Could you check a few things on this model? Use its own coordinates, in mm. A direction names the side the tool comes from. Give positions to 0.01 mm unless a question says otherwise; leave off trailing zeros. Loops run counter-clockwise (first coordinate to the right, second up) from the corner with the lowest first, then second, coordinate; pieces in that order, holes last. Notation, with made-up numbers: (47.25, 34.5) - (61.25, 34.5) arc R36 ccw to (61.25, 72.5) - close; hole circle Ø10 at (5, 56). An arc over 180 degrees is marked (long way). One line per item, written item: value. Start each with the question number.
Q1. I'm going to push flat-ended pins straight in: P1, Ø18, axis at x = 1.5, y = 18.5, coming from the +Z side; P2, Ø0.8, axis at x = -79, y = 0.5, coming from the -Z side; P3, Ø5, axis at x = -66, z = 0, coming from the +Y side. Where does each tip first touch, or does it pass through?
Q2. I want a section at D-D (y = 7). Please give me the cut outline in (x, z), then the cut area to 3 significant figures.
Q3. For faces 1 (the face through (-1.306, 5.572, 58.065)), 2 (the face through (-1, 1, -1)), 3 (the face through (-94.5, 10.6, -55)), 4 (the face through (94.6, 10.6, -55)), 5 (the face through (-94, 20, 1)), which set-ups out of +Z, -Z, +X, -X, +Y, -Y let a thin tool reach every point of the face, with its end or its side?
Q4. I want a section at C-C (x = 66). Please give me the cut outline in (y, z).
Q5. I want a section at B-B (z = 50). Please give me the cut outline in (x, y), then the cut area to 3 significant figures.
Q6. If I drill on line 1 (X direction, y = 36, z = -18); line 2 (Y direction, x = -69, z = -4); line 3 (Z direction, x = 42, y = 36.5), over which ranges is the centre line in solid material (lowest first)? Write a range as from..to.
Q7. I want a section at A-A (y = 31.5). Please give me the cut outline in (x, z).
Q8. If we mould it in two halves opening along X, with no side actions, what happens to faces 6 (the face through (1, 20, -55.737)), 7 (the face through (-93.263, 5, 58)), 8 (the face through (82.41, 0.49, -52.38))? For each: released by +X, released by -X, zero draft, split by the parting line, or undercut.
```python
from build123d import *

# Parameters (mm, degrees)
SKETCH2_W                    = 190
SKETCH2_H                    = 110
BASE_FLANGE1_DEPTH           = 1
EDGE_FLANGE1_STRIP_W         = 5.4732
EDGE_FLANGE1_STRIP_H         = 1
EDGE_FLANGE1_STRIP_CUT_DEPTH = 110
EDGE_FLANGE1_DEPTH           = 110
SKETCH16_R                   = 2.25
CUT_EXTRUDE1_DEPTH           = 117.163677628
SKETCH17_W                   = 10
SKETCH17_H                   = 25
CUT_EXTRUDE2_DEPTH           = 117.163677628
EDGE_FLANGE2_DEPTH           = 142
EDGE_FLANGE3_DEPTH           = 186.5268
SKETCH29_R                   = 2.25
CUT_EXTRUDE3_DEPTH           = 204.225548722
SKETCH30_R                   = 2.25
CUT_EXTRUDE4_DEPTH           = 120.271218881


# Sheet-metal steps are written as plain solids
with BuildPart() as part:
    # Sketch2 → Base-Flange1 (new body)
    with BuildSketch(Plane(origin=(0, 0, 0), x_dir=(1, 0, 0), z_dir=(0, 1, 0))):
        Rectangle(SKETCH2_W, SKETCH2_H)
    extrude(amount=BASE_FLANGE1_DEPTH)

    # Edge-Flange1 strip (across the edge) → Edge-Flange1 strip cut (cut)
    with BuildSketch(Plane(origin=(95, 1, 55), x_dir=(-1, 0, 0), z_dir=(0, 0, -1))):
        with Locations((-1, -0.5)):
            Rectangle(EDGE_FLANGE1_STRIP_W, EDGE_FLANGE1_STRIP_H)
    edge_flange1_strip_cut = extrude(amount=EDGE_FLANGE1_STRIP_CUT_DEPTH, mode=Mode.SUBTRACT)

    # Edge-Flange1 section (across the edge) → Edge-Flange1 (add)
    with BuildSketch(Plane(origin=(95, 1, 55), x_dir=(-1, 0, 0), z_dir=(0, 0, -1))):
        with BuildLine():
            Line((0, 0.7366), (0, 37))
            Line((0, 37), (1, 37))
            Line((1, 37), (1, 0.7366))
            ThreePointArc((1, 0.7366), (1.215745145, 0.215745145), (1.7366, 0))
            Line((1.7366, 0), (1.7366, -1))
            ThreePointArc((1.7366, -1), (0.508638364, -0.491361636), (0, 0.7366))
        make_face()
    edge_flange1 = extrude(amount=EDGE_FLANGE1_DEPTH)

    # Mirror1: Edge-Flange1 strip cut, Edge-Flange1 across plane
    add(edge_flange1_strip_cut.mirror(Plane(origin=(0, 0, 0), x_dir=(0, 0, 1), z_dir=(1, 0, 0))), mode=Mode.SUBTRACT)
    add(edge_flange1.mirror(Plane(origin=(0, 0, 0), x_dir=(0, 0, 1), z_dir=(1, 0, 0))))

    # Sketch16 → Cut-Extrude1 (cut, through all)
    with BuildSketch(Plane.XZ):
        with Locations(Location((-55, 0, 0), (0, 0, 270))):
            Circle(SKETCH16_R)
        with Locations(Location((55, 0, 0), (0, 0, 270))):
            Circle(SKETCH16_R)
        with Locations(Location((66, 0, 0), (0, 0, 270))):
            Circle(SKETCH16_R)
        with Locations(Location((-66, 0, 0), (0, 0, 270))):
            Circle(SKETCH16_R)
    extrude(amount=-CUT_EXTRUDE1_DEPTH, mode=Mode.SUBTRACT)

    # Sketch17 → Cut-Extrude2 (cut, through all)
    with BuildSketch(Plane.XZ):
        with Locations((-79, 0)):
            Rectangle(SKETCH17_W, SKETCH17_H)
    cut_extrude2 = extrude(amount=-CUT_EXTRUDE2_DEPTH, mode=Mode.SUBTRACT)

    # Mirror2: Cut-Extrude2 across plane
    add(cut_extrude2.mirror(Plane(origin=(0, 0, 0), x_dir=(0, 0, 1), z_dir=(1, 0, 0))), mode=Mode.SUBTRACT)

    # Edge-Flange2 section (across the edge) → Edge-Flange2 (add)
    with BuildSketch(Plane(origin=(71, 1, -55.7366), x_dir=(0, 0, 1), z_dir=(-1, 0, 0))):
        with BuildLine():
            Line((-1, 0.7366), (-1, 37))
            Line((-1, 37), (0, 37))
            Line((0, 37), (0, 0.7366))
            ThreePointArc((0, 0.7366), (0.215745145, 0.215745145), (0.7366, 0))
            Line((0.7366, 0), (0.7366, -1))
            ThreePointArc((0.7366, -1), (-0.491361636, -0.491361636), (-1, 0.7366))
        make_face()
    extrude(amount=EDGE_FLANGE2_DEPTH)

    # Edge-Flange3 section (across the edge) → Edge-Flange3 (add)
    with BuildSketch(Plane(origin=(-93.2634, 1, 55.425276208), x_dir=(0, 0.5000000000000041, -0.8660254037844364), z_dir=(1, 0, 0))):
        with BuildLine():
            Line((-1, 0.425276208), (-1, 10))
            Line((-1, 10), (0, 10))
            Line((0, 10), (0, 0.425276208))
            ThreePointArc((0, 0.425276208), (0.098685688, 0.056976208), (0.3683, -0.212638104))
            Line((0.3683, -0.212638104), (-0.1317, -1.078663508))
            ThreePointArc((-0.1317, -1.078663508), (-0.767339716, -0.443023792), (-1, 0.425276208))
        make_face()
    extrude(amount=EDGE_FLANGE3_DEPTH)

    # Sketch29 → Cut-Extrude3 (cut, through all)
    with BuildSketch(Plane.ZY.offset(95)):
        with Locations(Location((50, 19.8683, 0), (0, 0, 270))):
            Circle(SKETCH29_R)
    extrude(amount=-CUT_EXTRUDE3_DEPTH, mode=Mode.SUBTRACT)

    # Sketch30 → Cut-Extrude4 (cut, through all)
    with BuildSketch(Plane.XZ):
        with Locations(Location((81.73, -39.2366, 0), (0, 0, 270))):
            Circle(SKETCH30_R)
        with Locations(Location((81.73, -50.2366, 0), (0, 0, 270))):
            Circle(SKETCH30_R)
        with Locations(Location((-81.73, -39.2366, 0), (0, 0, 270))):
            Circle(SKETCH30_R)
        with Locations(Location((-81.73, -50.2366, 0), (0, 0, 270))):
            Circle(SKETCH30_R)
    extrude(amount=-CUT_EXTRUDE4_DEPTH, mode=Mode.SUBTRACT)


solid = part.part
```
Worked answers:
1. P1: stops at z = 60.7
1. P2: stops at z = -55
1. P3: stops at y = 1
2. outline: (-95, -55) - (-94, -55) - (-94, 55) - (-95, 55) - close; (-93.26, 58.89) - (93.26, 58.89) - (93.26, 60.04) - (-93.26, 60.04) - close; (-71, -56.74) - (71, -56.74) - (71, -55.74) - (-71, -55.74) - close; (94, -55) - (95, -55) - (95, 55) - (94, 55) - close
2. area: 577 mm²
3. face 1: +X, -X, +Y
3. face 2: +Y
3. face 3: -Z, -X, +Y, -Y
3. face 4: -Z, +X, +Y, -Y
3. face 5: +Z, -Z, +Y
4. outline: (0, -55) arc R1.74 ccw to (1.74, -56.74) - (38, -56.74) - (38, -55.74) - (1.74, -55.74) arc R0.74 cw to (1, -55) - (1, -2.25) - (0, -2.25) - close; (0, 2.25) - (1, 2.25) - (1, 55) arc R0.74 cw to (1.37, 55.64) - (9.66, 60.43) - (9.16, 61.29) - (0.87, 56.5) arc R1.74 ccw to (0, 55) - close
5. outline: (-95, 1.74) arc R1.74 ccw to (-93.26, 0) - (93.26, 0) arc R1.74 ccw to (95, 1.74) - (95, 17.62) - (94, 17.62) - (94, 1.74) arc R0.74 cw to (93.26, 1) - (-93.26, 1) arc R0.74 cw to (-94, 1.74) - (-94, 17.62) - (-95, 17.62) - close; (-95, 22.12) - (-94, 22.12) - (-94, 38) - (-95, 38) - close; (94, 22.12) - (95, 22.12) - (95, 38) - (94, 38) - close
5. area: 254 mm²
6. line 1: x = -95..-94, 94..95
6. line 2: y = 0..1
6. line 3: z = -56.74..-55.74
7. outline: (-95, -55) - (-94, -55) - (-94, 55) - (-95, 55) - close; (-71, -56.74) - (71, -56.74) - (71, -55.74) - (-71, -55.74) - close; (94, -55) - (95, -55) - (95, 55) - (94, 55) - close
8. face 6: zero draft
8. face 7: released by -X
8. face 8: undercut
